from build123d import *

# Parameters (mm, degrees)
F1_DEPTH = 500


with BuildPart() as f1:
    # F0 (on Front) → F1 (new body)
    with BuildSketch(Plane.XZ):
        with BuildLine():
            ThreePointArc((0, -2.45), (-1.732412, -1.732412), (-2.45, 0))
            Line((-2.45, 0), (-5.1, 0))
            Line((-5.1, 0), (-5.1, -2.508831))
            ThreePointArc((-5.1, -2.508831), (-5.290301, -3.46554), (-5.832233, -4.276598))
            Line((-5.832233, -4.276598), (-10.823402, -9.267767))
            ThreePointArc((-10.823402, -9.267767), (-11.63446, -9.809699), (-12.591169, -10))
            Line((-12.591169, -10), (-13, -10))
            ThreePointArc((-13, -10), (-13.353553, -9.853553), (-13.5, -9.5))
            Line((-13.5, -9.5), (-13.5, -6.4))
            ThreePointArc((-13.5, -6.4), (-13.353553, -6.046447), (-13, -5.9))
            Line((-13, -5.9), (-12.6, -5.9))
            ThreePointArc((-12.6, -5.9), (-12.246447, -5.753553), (-12.1, -5.4))
            Line((-12.1, -5.4), (-12.1, -3.5))
            ThreePointArc((-12.1, -3.5), (-12.246447, -3.146447), (-12.6, -3))
            Line((-12.6, -3), (-14.5, -3))
            ThreePointArc((-14.5, -3), (-14.853553, -3.146447), (-15, -3.5))
            Line((-15, -3.5), (-15, -12))
            ThreePointArc((-15, -12), (-14.12132, -14.12132), (-12, -15))
            Line((-12, -15), (-3.5, -15))
            ThreePointArc((-3.5, -15), (-3.146447, -14.853553), (-3, -14.5))
            Line((-3, -14.5), (-3, -12.6))
            ThreePointArc((-3, -12.6), (-3.146447, -12.246447), (-3.5, -12.1))
            Line((-3.5, -12.1), (-5.4, -12.1))
            ThreePointArc((-5.4, -12.1), (-5.753553, -12.246447), (-5.9, -12.6))
            Line((-5.9, -12.6), (-5.9, -13))
            ThreePointArc((-5.9, -13), (-6.046447, -13.353553), (-6.4, -13.5))
            Line((-6.4, -13.5), (-9.5, -13.5))
            ThreePointArc((-9.5, -13.5), (-9.853553, -13.353553), (-10, -13))
            Line((-10, -13), (-10, -12.591169))
            ThreePointArc((-10, -12.591169), (-9.809699, -11.63446), (-9.267767, -10.823402))
            Line((-9.267767, -10.823402), (-4.276598, -5.832233))
            ThreePointArc((-4.276598, -5.832233), (-3.46554, -5.290301), (-2.508831, -5.1))
            Line((-2.508831, -5.1), (0, -5.1))
            Line((0, -5.1), (0, -2.45))
        make_face()
        with BuildLine():
            Line((-11.5, -13.5), (-12.5, -13.5))
            ThreePointArc((-12.5, -13.5), (-13.207107, -13.207107), (-13.5, -12.5))
            Line((-13.5, -12.5), (-13.5, -11.5))
            ThreePointArc((-13.5, -11.5), (-13.353553, -11.146447), (-13, -11))
            Line((-13, -11), (-11.5, -11))
            ThreePointArc((-11.5, -11), (-11.146447, -11.146447), (-11, -11.5))
            Line((-11, -11.5), (-11, -13))
            ThreePointArc((-11, -13), (-11.146447, -13.353553), (-11.5, -13.5))
        make_face(mode=Mode.SUBTRACT)
    extrude(amount=F1_DEPTH)

    # F2: F1 across plane


with BuildPart() as f1_1:
    add(f1.part)
    add(f1.part.mirror(Plane.YZ))

    # F3: F1 across plane


with BuildPart() as f1_2:
    add(f1_1.part)
    add(f1_1.part.mirror(Plane.XY))


solid = f1_2.part
Geometry: final body of the model. Coordinates: model frame, mm. Round coordinates to 2 decimals unless told otherwise and drop trailing zeros. One line per question, with ' | ' between items.
(1) Contact query for a flat-ended pin moving along its axis: P1, Ø2.5, axis at x = 0, y = -372.5, coming from the +Z side. Output: stop coordinate, or through.
Check result:
P1: stops at z = 5.1
(2) Material intervals for line 1 along Z through (x, y) = (12.5, -425); line 2 along Z through (x, y) = (8, -437), sorted ascending. Write a range as from..to.
Check result:
line 1: z = -14.96..-13.5, -11..-10, -5.89..-3.01, 3.01..5.89, 10..11, 13.5..14.96 | line 2: z = -15..-13.5, -9.56..-6.44, 6.44..9.56, 13.5..15
(3) Cut plane A-A on y = -447.5. Give the number of separate pieces and of enclosed holes in the cut face, plus the area to 3 significant figures.
Check result:
separate pieces: 1 | enclosed holes: 5 | area: 343 mm2
